```python
from build123d import *

# Parameters (mm, degrees)
ESBO_O1_R                = 6
RESSALTO_EXTRUS_O1_DEPTH = 1
ESBO_O2_R                = 3.5
RESSALTO_EXTRUS_O2_DEPTH = 12
CORTE_EXTRUS_O1_START    = -2
ESBO_O3_R                = 3.5
ESBO_O3_R_2              = 3
CORTE_EXTRUS_O1_DEPTH    = 1


with BuildPart() as part:
    # Esboço1 → Ressalto-extrusão1 (new body)
    with BuildSketch(Plane(origin=(0, 0, 0), x_dir=(1, 0, 0), z_dir=(0, 1, 0))):
        with Locations(Location((0, 0, 0), (0, 0, 270))):
            Circle(ESBO_O1_R)
    extrude(amount=RESSALTO_EXTRUS_O1_DEPTH)

    # Esboço2 → Ressalto-extrusão2 (add)
    with BuildSketch(Plane(origin=(0, 1, 0), x_dir=(1, 0, 0), z_dir=(0, 1, 0))):
        with Locations(Location((0, 0, 0), (0, 0, 270))):
            Circle(ESBO_O2_R)
    extrude(amount=RESSALTO_EXTRUS_O2_DEPTH)

    # Esboço3 → Corte-extrusão1 (cut)
    with BuildSketch(Plane(origin=(0, 13, 0), x_dir=(1, 0, 0), z_dir=(0, 1, 0)).offset(CORTE_EXTRUS_O1_START)):
        with Locations(Location((0, 0, 0), (0, 0, 270))):
            Circle(ESBO_O3_R)
        with Locations(Location((0, 0, 0), (0, 0, 270))):
            Circle(ESBO_O3_R_2, mode=Mode.SUBTRACT)
    extrude(amount=CORTE_EXTRUS_O1_DEPTH, mode=Mode.SUBTRACT)


solid = part.part
```
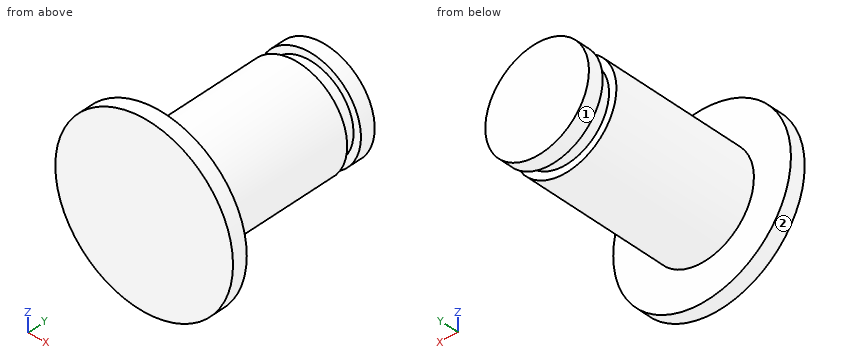
Verification items for the finished model (mm, model axes). Face numbers are marked on the shaded views. A direction names the side the tool comes from. Coordinates: 2 decimals unless noted, no trailing zeros. Write each loop counter-clockwise with the first axis right and the second up, starting at its lowest first coordinate (ties: lowest second). Pieces come first, ordered by that corner, then holes. Notation, with made-up numbers: M -25.75,42.5 L 17.25,42.5 A14 ccw 17.25,64.5 Z; hole C 39,45.5 d7. An arc over 180 degrees is marked long. Answer as a JSON object with one key per item and string values. Group by question number.
(1) Tool access check on the marked faces 1 and 2. Record the directions out of +Z, -Z, +X, -X, +Y, -Y that give a thin tool (end or side, any length) a straight path to the whole face; none if there is none.
(2) Material ranges on line 1 (Y direction, x = 2.5, z = -2); line 2 (Y direction, x = 2.5, z = -3); line 3 (X direction, y = 11.25, z = 0.5), recorded low to high.
(3) Gauge pin test, flat ends, axial feed: pin 1 (4 mm diameter, centred on x = 3, y = 6, fed in from +Z); pin 2 (4 mm diameter, centred on y = 5, z = 0, fed in from -X); pin 3 (6 mm diameter, centred on y = 9, z = 0, fed in from +X). Record the tip position at first contact, or that the pin passes through.
(4) Cross-section at A-A, the plane z = 0. Record the cut outline in (x, y), and give its area (3 significant figures).
(5) Cross-section at C-C, the plane x = -3.25. Record the cut outline in (y, z), and give its area (3 significant figures).
(6) Cross-section at B-B, the plane x = 0. Record the cut outline in (y, z), and give its area (3 significant figures).
(7) Cross-section at D-D, the plane y = 3.25. Record the cut outline in (x, z), and give its area (3 significant figures).
Reply:
{
 "1": {"face 1": "+Y", "face 2": "+Y, -Y"},
 "2": {"line 1": "0 to 11, 12 to 13", "line 2": "0 to 1", "line 3": "-2.96 to 2.96"},
 "3": {"pin 1": "z = 3.35", "pin 2": "x = -3.5", "pin 3": "x = 3.5"},
 "4": {"outline": "M -6,0 L 6,0 L 6,1 L 3.5,1 L 3.5,11 L 3,11 L 3,12 L 3.5,12 L 3.5,13 L -3.5,13 L -3.5,12 L -3,12 L -3,11 L -3.5,11 L -3.5,1 L -6,1 Z", "area": "95.0 mm²"},
 "5": {"outline": "M 0,-5.04 L 1,-5.04 L 1,-1.3 L 11,-1.3 L 11,1.3 L 1,1.3 L 1,5.04 L 0,5.04 Z; M 12,-1.3 L 13,-1.3 L 13,1.3 L 12,1.3 Z", "area": "38.7 mm²"},
 "6": {"outline": "M 0,-6 L 1,-6 L 1,-3.5 L 11,-3.5 L 11,-3 L 12,-3 L 12,-3.5 L 13,-3.5 L 13,3.5 L 12,3.5 L 12,3 L 11,3 L 11,3.5 L 1,3.5 L 1,6 L 0,6 Z", "area": "95.0 mm²"},
 "7": {"outline": "C 0,0 d7", "area": "38.5 mm²"}
}
